```python
from build123d import *

# Parameters (mm, degrees)
F0_W     = 6
F0_H     = 15
F1_DEPTH = 3
F2_T     = -0.2
F3_W     = 0.2
F3_H     = 14
F4_DEPTH = 2.8


with BuildPart() as f1:
    # F0 (on Top) → F1 (new body)
    with BuildSketch(Plane.XY):
        Rectangle(F0_W, F0_H)
    extrude(amount=F1_DEPTH)

    # F2
    f2_openings = [f1.faces().sort_by_distance(p)[0] for p in [
        (0, 0, 3),
    ]]
    offset(amount=F2_T, openings=f2_openings)

    # F3 (on face) → F4 (join)
    with BuildSketch(Plane.XY.offset(0.2)):
        with Locations((-1.903401, 0.3)):
            Rectangle(F3_W, F3_H)
    extrude(amount=F4_DEPTH)


solid = f1.part
```
Geometry check sheet. Reference: the model listing, model coordinates, mm. A direction names the side the tool comes from. Round coordinates to 2 decimals unless told otherwise and drop trailing zeros. Write each loop counter-clockwise with the first axis right and the second up, starting at its lowest first coordinate (ties: lowest second). Pieces come first, ordered by that corner, then holes. Notation, with made-up numbers: (20.5, -29.75) - (52.5, -29.75) arc R15 cw to (52.5, -7.75) - close; hole circle Ø10 at (21, 51). An arc over 180 degrees is marked (long way). Write each question's results on one line, items separated by ' | '.
(1) Depth check by flat-ended pin: pin 1 Ø1 at (x, y) = (0, -2) entering from +Z. Enter the tip coordinate at first touch or a pass-through.
Computed:
pin 1: stops at z = 0.2
(2) Sectioned sample at B-B, the plane y = -3. Enter the section's corners in (x, z).
Computed:
outline: (-3, 0) - (3, 0) - (3, 3) - (2.8, 3) - (2.8, 0.2) - (-1.8, 0.2) - (-1.8, 3) - (-2, 3) - (-2, 0.2) - (-2.8, 0.2) - (-2.8, 3) - (-3, 3) - close
(3) Sectioned sample at A-A, the plane z = 0.35. Enter the section's corners in (x, y), plus the area to 3 significant figures.
Computed:
outline: (-3, -7.5) - (3, -7.5) - (3, 7.5) - (-3, 7.5) - close; hole (-2.8, -7.3) - (2.8, -7.3) - (2.8, 7.3) - (-1.8, 7.3) - (-1.8, -6.7) - (-2, -6.7) - (-2, 7.3) - (-2.8, 7.3) - close | area: 11.0 mm^2
(4) Thickness scan on probe 1 along X at (y, z) = (1.75, 2.9); probe 2 along Y at (x, z) = (2.4, 0.6); probe 3 along X at (y, z) = (-7, 2.7). Record the ranges inside material, lowest first. Write a range as from..to.
Computed:
probe 1: x = -3..-2.8, -2..-1.8, 2.8..3 | probe 2: y = -7.5..-7.3, 7.3..7.5 | probe 3: x = -3..-2.8, 2.8..3
(5) Draft check along X on faces 1 (the face through (2.8, 0, 2)), 2 (the face through (0, -7.5, 1)), 3 (the face through (-3, 0, 1)), 4 (the face through (-1.803, 0, 2)). Enter one of: pulls with the +X half, pulls with the -X half, needs draft (parallel to the pull), parting line crosses it, or undercut.
Computed:
face 1: undercut | face 2: needs draft | face 3: pulls with the -X half | face 4: undercut
(6) Sectioned sample at C-C, the plane x = -0.55. Enter the section's corners in (y, z), plus the area to 3 significant figures.
Computed:
outline: (-7.5, 0) - (7.5, 0) - (7.5, 3) - (7.3, 3) - (7.3, 0.2) - (-7.3, 0.2) - (-7.3, 3) - (-7.5, 3) - close | area: 4.12 mm^2
(7) Set-up check for faces 5 (the face through (3, 0, 1)), 6 (the face through (0, -7.3, 2)): record each of +Z, -Z, +X, -X, +Y, -Y from which the full face is reachable in a straight line by a thin tool's end or side.
Computed:
face 5: +Z, -Z, +X, +Y, -Y | face 6: +Z
